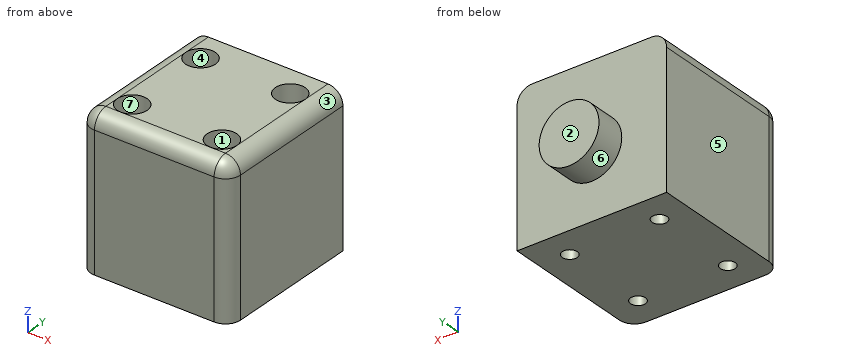
from build123d import *

# Parameters (mm, degrees)
F0_W     = 50
F0_H     = 50
F0_R     = 5
F0_R_2   = 2.5
F1_DEPTH = 50
F2_START = 10
F2_DEPTH = 40
F3_R     = 4.99999
F4_R     = 10
F5_DEPTH = 10


# Not quite as in the source:
# - a fillet or chamfer is up to 0.001 mm smaller than in the source, because OpenCascade refuses the exact size


with BuildPart() as f1:
    # F0 (on Top) → F1 (new body)
    with BuildSketch(Plane.XY):
        Rectangle(F0_W, F0_H)
        with Locations((-15, -15)):
            Circle(F0_R, mode=Mode.SUBTRACT)
        with Locations((15, -15)):
            Circle(F0_R, mode=Mode.SUBTRACT)
        with Locations((-15, 15)):
            Circle(F0_R, mode=Mode.SUBTRACT)
        with Locations((15, 15)):
            Circle(F0_R, mode=Mode.SUBTRACT)
        with Locations((-15, -15)):
            Circle(F0_R)
        with Locations((-15, -15)):
            Circle(F0_R_2, mode=Mode.SUBTRACT)
        with Locations((-15, 15)):
            Circle(F0_R)
        with Locations((-15, 15)):
            Circle(F0_R_2, mode=Mode.SUBTRACT)
        with Locations((15, 15)):
            Circle(F0_R)
        with Locations((15, 15)):
            Circle(F0_R_2, mode=Mode.SUBTRACT)
        with Locations((15, -15)):
            Circle(F0_R)
        with Locations((15, -15)):
            Circle(F0_R_2, mode=Mode.SUBTRACT)
    extrude(amount=F1_DEPTH)

    # F0 (on Top) → F2 (cut)
    with BuildSketch(Plane.XY.offset(F2_START)):
        with Locations((-15, -15)):
            Circle(F0_R)
        with Locations((-15, -15)):
            Circle(F0_R_2, mode=Mode.SUBTRACT)
        with Locations((-15, 15)):
            Circle(F0_R)
        with Locations((-15, 15)):
            Circle(F0_R_2, mode=Mode.SUBTRACT)
        with Locations((15, -15)):
            Circle(F0_R)
        with Locations((15, -15)):
            Circle(F0_R_2, mode=Mode.SUBTRACT)
        with Locations((15, 15)):
            Circle(F0_R)
        with Locations((15, 15)):
            Circle(F0_R_2, mode=Mode.SUBTRACT)
    extrude(amount=F2_DEPTH, mode=Mode.SUBTRACT)

    # F3 (radius 5 in the source; OpenCascade refuses exactly that, so slightly less here)
    f3_edges = [f1.edges().sort_by_distance(p)[0] for p in [
        (-25, -25, 25),
        (25, -25, 25),
        (0, -25, 50),
        (-25, 0, 50),
        (25, 0, 50),
    ]]
    fillet(f3_edges, radius=F3_R)

    # F4 (on face) → F5 (join)
    with BuildSketch(Plane(origin=(0, 25, 0), x_dir=(-1, 0, 0), z_dir=(0, 1, 0))):
        with Locations((0, 22.5)):
            Circle(F4_R)
    extrude(amount=F5_DEPTH)


solid = f1.part
Verification items for the finished model (mm, model axes). Face numbers are marked on the shaded views. A direction names the side the tool comes from. Give positions to 0.01 mm unless a question says otherwise; leave off trailing zeros. Write each loop counter-clockwise with the first axis right and the second up, starting at its lowest first coordinate (ties: lowest second). Pieces come first, ordered by that corner, then holes. Notation, with made-up numbers: (-20, 47) -> (28, 47) arc R29 cw to (28, 83) -> close; hole circle Ø10 at (3, 81.5). An arc over 180 degrees is marked (long way). Use CSV: the item, a comma, the result in double quotes.
(1) Sectioned sample at D-D (x = 11). Record the cut outline in (y, z).
Derived:
outline,"(-25, 0) -> (25, 0) -> (25, 50) -> (18, 50) -> (18, 10) -> (12, 10) -> (12, 50) -> (-12, 50) -> (-12, 10) -> (-18, 10) -> (-18, 50) -> (-20, 50) arc R5 ccw to (-25, 45) -> close"
(2) Set-up check for the marked faces 5, 6 and 7: record each of +Z, -Z, +X, -X, +Y, -Y from which the full face is reachable in a straight line by a thin tool's end or side.
Derived:
face 5,"+Z, -Z, -X, +Y, -Y"
face 6,"+Y"
face 7,"+Z"
(3) Sectioned sample at C-C (z = 22.5). Record the cut outline in (x, y), plus the area to 3 significant figures.
Derived:
outline,"(-25, -20) arc R5 ccw to (-20, -25) -> (20, -25) arc R5 ccw to (25, -20) -> (25, 25) -> (10, 25) -> (10, 35) -> (-10, 35) -> (-10, 25) -> (-25, 25) -> close; hole circle Ø10 at (-15, -15); hole circle Ø10 at (-15, 15); hole circle Ø10 at (15, -15); hole circle Ø10 at (15, 15)"
area,"2,380 mm^2"
(4) Go/stop test with flat-tipped pins: pin 1 (6 mm diameter, centred on x = -15, y = 15, fed in from +Z); pin 2 (4.5 mm diameter, centred on x = -15, y = 15, fed in from +Z). Record where each tip stops, or that it passes through.
Derived:
pin 1,"stops at z = 10"
pin 2,"passes through"
(5) Sectioned sample at A-A (x = -15). Give the number of separate pieces and of enclosed holes in the cut face, plus the area to 3 significant figures.
Derived:
separate pieces,"3"
enclosed holes,"0"
area,"1,590 mm^2"
(6) Release check for a two-part mould opening along X. For the marked faces 1, 2, 3 and 4 record: +X half, -X half, draft (parallel to the pull), parting line (faces both ways), or undercut.
Derived:
face 1,"undercut"
face 2,"draft"
face 3,"+X half"
face 4,"undercut"
(7) Material ranges on L1, parallel to Y at x = 15, z = 2; L2, parallel to Y at x = -15, z = 25; L3, parallel to X at y = -18.5, z = 12.5, recorded low to high.
Derived:
L1,"y = -25 to -17.5, -12.5 to 12.5, 17.5 to 25"
L2,"y = -25 to -20, -10 to 10, 20 to 25"
L3,"x = -25 to -18.57, -11.43 to 11.43, 18.57 to 25"
